CAD build for the part. Positions are in the model's coordinates, mm. Face numbers are marked on the shaded views. A direction names the side the tool comes from. Coordinates: 2 decimals unless noted, no trailing zeros. Order: outer loops, then holes, each group sorted by start corner. A loop starts at its lowest first (then second) coordinate and runs counter-clockwise, first axis right, second up.
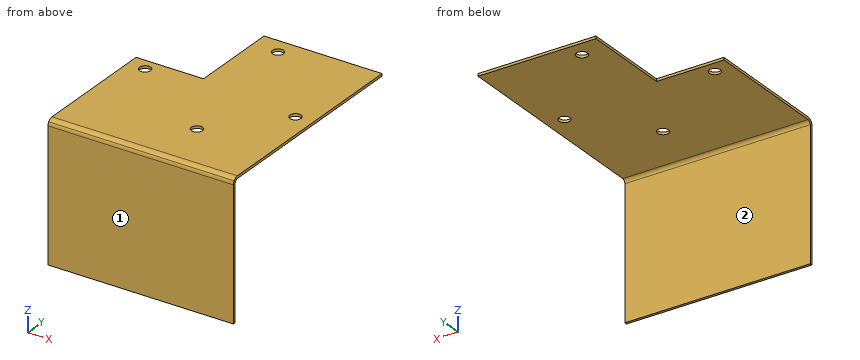
from build123d import *

# Parameters (mm, degrees)
ESBO_O1_W                   = 110
ESBO_O1_H                   = 210
RESSALTO_EXTRUS_O1_DEPTH    = 1.5
FURO_COM_FOLGA_DE_M62_D     = 6.6
FURO_COM_FOLGA_DE_M62_DEPTH = 10
FURO_COM_FOLGA_DE_M62_TIP   = 1.982840043
ESBO_O4_W                   = 40
ESBO_O4_H                   = 53.5
CORTE_EXTRUS_O1_DEPTH       = 119.542186584
DOBRA_START                 = -55
DOBRA_ESBO_ADA1_DEPTH       = 110
DOBRA_ESBO_ADA1_2_DEPTH     = 110


# Read off the part's stored shape, not the designer's step: Transforma__o de esbo_o2
with BuildPart() as part:
    # Esboço1 → Ressalto-extrusão1 (new body)
    with BuildSketch(Plane.XY):
        Rectangle(ESBO_O1_W, ESBO_O1_H)
    extrude(amount=RESSALTO_EXTRUS_O1_DEPTH)

    # Furo com folga de M62
    with Locations(Plane.XY.offset(1.5)):
        with Locations((0, 95), (-44.6, 44), (44.6, 44), (11.3, 6.5)):
            Hole(FURO_COM_FOLGA_DE_M62_D / 2, depth=FURO_COM_FOLGA_DE_M62_DEPTH)
            with Locations((0, 0, -(FURO_COM_FOLGA_DE_M62_DEPTH + FURO_COM_FOLGA_DE_M62_TIP / 2))):  # 118° drill point
                Cone(0, FURO_COM_FOLGA_DE_M62_D / 2, FURO_COM_FOLGA_DE_M62_TIP, mode=Mode.SUBTRACT)

    # Esboço4 → Corte-extrusão1 (cut, through all)
    with BuildSketch(Plane.XY.offset(1.5)):
        with Locations((-35, 78.25)):
            Rectangle(ESBO_O4_W, ESBO_O4_H)
    extrude(amount=-CORTE_EXTRUS_O1_DEPTH, mode=Mode.SUBTRACT)

    # Dobra esboçada1 outline → Dobra esboçada1 (cut)
    with BuildSketch(Plane.YZ.offset(DOBRA_START)):
        with BuildLine():
            Line((-105, 0), (-25.712436374, 0))
            ThreePointArc((-25.712436374, 0), (-24.460340225, 1.102418411), (-22.840155051, 1.5))
            Line((-22.840155051, 1.5), (-105, 1.5))
            Line((-105, 1.5), (-105, 0))
        make_face()
    extrude(amount=DOBRA_ESBO_ADA1_DEPTH, mode=Mode.SUBTRACT)

    # Dobra esbo_ada1 2 outline → Dobra esbo_ada1 2 (add)
    with BuildSketch(Plane.YZ.offset(DOBRA_START)):
        with BuildLine():
            ThreePointArc((-25.712436374, 0), (-26.179540071, -0.951902827), (-26.340155051, -2))
            Line((-26.340155051, -2), (-26.340155051, -79.840155051))
            Line((-26.340155051, -79.840155051), (-24.840155051, -79.840155051))
            Line((-24.840155051, -79.840155051), (-24.840155051, -2))
            ThreePointArc((-24.840155051, -2), (-24.254368613, -0.585786438), (-22.840155051, 0))
            Line((-22.840155051, 0), (-25.712436374, 0))
        make_face()
    extrude(amount=DOBRA_ESBO_ADA1_2_DEPTH)


solid = part.part
1) Slice it at D-D (x = 20.5). List the corners of the cut face in (y, z), plus the area to 3 significant figures.
2) Slice it at C-C (y = 44). List the corners of the cut face in (x, z), plus the area to 3 significant figures.
3) Drill centre lines: probe 1 along Y at (x, z) = (-17, -37); probe 2 along Z at (x, y) = (5.5, 85); probe 3 along Y at (x, z) = (11.3, 0.7). Where is each one in solid material? Low to high.
4) Slice it at B-B (x = 44.6). List the corners of the cut face in (y, z).
5) Slice it at A-A (y = 6.5). List the corners of the cut face in (x, z), plus the area to 3 significant figures.
6) Which spindle directions (+Z, -Z, +X, -X, +Y, -Y) get a long thin tool onto all of the face, cutting with end or side? Do the marked faces 1 and 2. Say none if no direction does.
7) Pin check, flat tips, straight feed: P1, Ø7.5, axis at x = 11.3, y = 6.5, coming from the -Z side; P2, Ø1.6, axis at x = -25.5, z = 1, coming from the +Y side; P3, Ø0.8, axis at y = 68.5, z = 0.5, coming from the -X side; P4, Ø4, axis at x = 0, y = 95, coming from the -Z side. Stop position of each tip, or through.
Worked out:
1. outline: (-26.34, -79.84) - (-24.84, -79.84) - (-24.84, -2) arc R2 cw to (-22.84, 0) - (105, 0) - (105, 1.5) - (-22.84, 1.5) arc R3.5 ccw to (-26.34, -2) - close
1. area: 315 mm2
2. outline: (-55, 0) - (-47.9, 0) - (-47.9, 1.5) - (-55, 1.5) - close; (-41.3, 0) - (41.3, 0) - (41.3, 1.5) - (-41.3, 1.5) - close; (47.9, 0) - (55, 0) - (55, 1.5) - (47.9, 1.5) - close
2. area: 145 mm2
3. probe 1: y = -26.34 to -24.84
3. probe 2: z = 0 to 1.5
3. probe 3: y = -25.07 to 3.2, 9.8 to 105
4. outline: (-26.34, -79.84) - (-24.84, -79.84) - (-24.84, -2) arc R2 cw to (-22.84, 0) - (40.7, 0) - (40.7, 1.5) - (-22.84, 1.5) arc R3.5 ccw to (-26.34, -2) - close; (47.3, 0) - (105, 0) - (105, 1.5) - (47.3, 1.5) - close
5. outline: (-55, 0) - (8, 0) - (8, 1.5) - (-55, 1.5) - close; (14.6, 0) - (55, 0) - (55, 1.5) - (14.6, 1.5) - close
5. area: 155 mm2
6. face 1: +Z, -Z, +X, -X, -Y
6. face 2: -Z, +X, -X, +Y
7. P1: stops at z = 0
7. P2: stops at y = 51.5
7. P3: stops at x = -15
7. P4: passes through
